Autodesk Inventor part; units mm, degrees
ref_plane "YZ Plane" through (0, 0, 0) normal (1, 0, 0) x (0, 1, 0)
ref_plane "XZ Plane" through (0, 0, 0) normal (0, 1, 0) x (-1, 0, 0)
ref_plane "XY Plane" through (0, 0, 0) normal (0, 0, 1) x (1, 0, 0)
sketch "Sketch1" plane through (0, 0, 0) normal (0, 0, 1) x (1, 0, 0)
  circle A0 centre (0, 0) radius 20
  dimension "d0" = 40
extrude "Extrusion1" add sketch "Sketch1" along normal blind 5
sketch "Sketch2" plane through (0, 0, 5) normal (0, 0, 1) x (1, 0, 0)
  circle A0 centre (0, 0) radius 2
  dimension "d3" = 4
extrude "Extrusion2" add sketch "Sketch2" along normal blind 12
sketch "Sketch3" plane through (0, 0, 17) normal (0, 0, 1) x (1, 0, 0)
  circle A0 centre (0, 0) radius 20
  dimension "d6" = 40
extrude "Extrusion3" add sketch "Sketch3" along normal blind 1
sketch "Sketch4" plane through (0, 0, 18) normal (0, 0, 1) x (1, 0, 0)
  circle A0 centre (0, 0) radius 1.1
  dimension "d9" = 2.2
extrude "Extrusion4" cut sketch "Sketch4" against normal through all
sketch "Sketch6" plane through (0, 0, 18) normal (0, 0, 1) x (1, 0, 0)
  circle A0 centre (0, 0) radius 2 construction
  circle A1 centre (-15.5, -10.6066) radius 0.4
  circle A2 centre (-2.5, 0) radius 0.4
  circle A3 centre (0, 0) radius 20
  dimension "d20" = 0.8
  dimension "d21" = 0.8
  dimension "d38" = 2.5
  dimension "d39" = 15.5
sketch "Sketch7" plane through (0, 0, 18) normal (0, 0, 1) x (1, 0, 0)
  point P0 (0, 0)
extrude "Extrusion5" cut sketch "Sketch6" against normal up to surface (1 mm away) contours A1 | A2
chamfer "Chamfer1" distance 0.4 angle 45 2 edges at (-2.9, 0, 18) (-15.9, -10.6066, 18)
sketch "Sketch11" plane through (0, 0, 0) normal (0, 0, -1) x (-1, 0, 0)
  circle A0 centre (0, 0) radius 20
  point P0 (-5, 26.5)
  point P1 (-5, -26.5)
  dimension "d40" = 26.5
  dimension "d41" = 5
  dimension "d42" = 5
  dimension "d43" = 26.5
hole "Hole3" at (5, -26.5, 0) at (5, 26.5, 0) direction (0, 0, 1) diameter 1.567 end through all
sketch "Sketch12" plane through (0, 0, 0) normal (0, 0, -1) x (-1, 0, 0)
  point P0 (0, 0)
  point P1 (5, 0)
  point P2 (-5, 0)
  dimension "d55" = 5
  dimension "d56" = 5
hole "Hole4" at (-5, 0, 0) at (5, 0, 0) direction (0, 0, 1) diameter 2.459 depth 4.8
loft "Loft1" [suppressed]
properties part number "Bobbin_z"
Can you work these out from the model? Positions are in its coordinate system, mm. A direction names the side the tool comes from. Give positions to 0.01 mm unless a question says otherwise; leave off trailing zeros. Loops run counter-clockwise (first coordinate to the right, second up) from the corner with the lowest first, then second, coordinate; pieces in that order, holes last. Notation, with made-up numbers: (51, 4.25) - (79, 4.25) arc R22 ccw to (79, 29.25) - close; hole circle Ø9 at (86.5, 30). An arc over 180 degrees is marked (long way). One line per item, written item: value.
(1) I need wall thicknesses on line 1 along Z through (x, y) = (-3, -15.5); line 2 along Y through (x, z) = (0, 8); line 3 along Y through (x, z) = (-2.5, 17.2). Which ranges of each line are inside material? Lowest first, please.
Verdict:
line 1: 0 to 5, 17 to 18
line 2: -2 to -1.1, 1.1 to 2
line 3: -19.84 to -0.4, 0.4 to 19.84
(2) If we mould it in two halves opening along Z, with no side actions, what happens to faces 1 (the face through (-4.336, 19.524, 2.465)), 2 (the face through (4, 0, 5)), 3 (the face through (5, 0, 4.8))? For each: released by +Z, released by -Z, zero draft, split by the parting line, or undercut.
Verdict:
face 1: zero draft
face 2: undercut
face 3: released by -Z
(3) If we section it at B-B, the plane z = 2: List the corners of the cut face in (x, y) for me, plus the area to 3 significant figures.
Verdict:
outline: circle Ø40 at (0, 0); hole circle Ø2.46 at (-5, 0); hole circle Ø2.2 at (0, 0); hole circle Ø2.46 at (5, 0)
area: 1,240 mm^2
(4) On a 3-axis mill with a long thin cutter (end or side, diameter ignored), from which of +Z, -Z, +X, -X, +Y, -Y can I reach the whole of each face in a straight line? I mean faces 4 (the face through (0, 2, 11)), 5 (the face through (-5, 0, 4.8)), 6 (the face through (1.05, 0.33, 9.13)). Say none if no direction works.
Verdict:
face 4: none
face 5: -Z
face 6: +Z, -Z
(5) If we section it at A-A, the plane y = 5.5: List the corners of the cut face in (x, z) for me.
Verdict:
outline: (-19.23, 0) - (19.23, 0) - (19.23, 5) - (-19.23, 5) - close; (-19.23, 17) - (19.23, 17) - (19.23, 18) - (-19.23, 18) - close
(6) If we section it at D-D, the plane y = -3: List the corners of the cut face in (x, z) for me, plus the area to 3 significant figures.
Verdict:
outline: (-19.77, 0) - (19.77, 0) - (19.77, 5) - (-19.77, 5) - close; (-19.77, 17) - (19.77, 17) - (19.77, 18) - (-19.77, 18) - close
area: 237 mm^2
(7) I'm going to push flat-ended pins straight in: pin 1 (5 mm diameter, centred on y = 7.5, z = 15.5, fed in from +X); pin 2 (3 mm diameter, centred on y = -2, z = 9.5, fed in from -X); pin 3 (1.5 mm diameter, centred on y = -1, z = 2, fed in from +X); pin 4 (3.5 mm diameter, centred on x = 0, y = 0, fed in from +Z). Where does each tip first touch, or does it pass through?
Verdict:
pin 1: x = 19.23
pin 2: x = -1.94
pin 3: x = 20
pin 4: z = 18
(8) If we section it at C-C, the plane x = 5: List the corners of the cut face in (y, z) for me, plus the area to 3 significant figures.
Verdict:
outline: (-19.36, 0) - (-1.23, 0) - (-1.23, 4.8) - (1.23, 4.8) - (1.23, 0) - (19.36, 0) - (19.36, 5) - (-19.36, 5) - close; (-19.36, 17) - (19.36, 17) - (19.36, 18) - (-19.36, 18) - close
area: 221 mm^2
